from build123d import *

# Parameters (mm, degrees)
SKIZZE1_R                            = 115
AUFSATZ_LINEAR_AUSTRAGEN1_DEPTH      = 730
AUFSATZ_LINEAR_AUSTRAGEN2_DEPTH      = 120
AUFSATZ_LINEAR_AUSTRAGEN2_DEPTH_BACK = 120
SKIZZE2_R                            = 21.686343762


with BuildPart() as part:
    # Skizze1 → Aufsatz-Linear austragen1 (new body)
    with BuildSketch(Plane.XY):
        with Locations(Location((0, 0, 0), (0, 0, 180))):
            Circle(SKIZZE1_R)
    extrude(amount=AUFSATZ_LINEAR_AUSTRAGEN1_DEPTH)

    # Skizze2 → Aufsatz-Linear austragen2 (add, two sides: drawn at the far end of the back side and taken through both)
    with BuildSketch(Plane(origin=(0, 0, 0), x_dir=(1, 0, 0), z_dir=(0, 1, 0)).offset(-AUFSATZ_LINEAR_AUSTRAGEN2_DEPTH_BACK)):
        with Locations(Location((0, -480, 0), (0, 0, 270))):
            Circle(SKIZZE2_R)
    extrude(amount=AUFSATZ_LINEAR_AUSTRAGEN2_DEPTH + AUFSATZ_LINEAR_AUSTRAGEN2_DEPTH_BACK)


solid = part.part
Input: part model. Units: mm. Frame: model coordinates. A direction names the side the tool comes from. Round coordinates to 2 decimals unless told otherwise and drop trailing zeros. Order: outer loops, then holes, each group sorted by start corner. A loop starts at its lowest first (then second) coordinate and runs counter-clockwise, first axis right, second up.
1. Cut plane B-B, the plane x = 0. Output: boundary loops of the cut face in (y, z), then the cut area to 3 significant figures.
The answers:
outline: (-120, 458.31) - (-115, 458.31) - (-115, 0) - (115, 0) - (115, 458.31) - (120, 458.31) - (120, 501.69) - (115, 501.69) - (115, 730) - (-115, 730) - (-115, 501.69) - (-120, 501.69) - close
area: 168,000 mm2
2. Material intervals for line 1 (Y direction, x = -0.5, z = 70); line 2 (Y direction, x = -89, z = 442.5); line 3 (X direction, y = -39, z = 257), sorted ascending.
The answers:
line 1: y = -115 to 115
line 2: y = -72.83 to 72.83
line 3: x = -108.19 to 108.19
3. Cut plane C-C, the plane y = 93. Output: boundary loops of the cut face in (x, z).
The answers:
outline: (-67.65, 0) - (67.65, 0) - (67.65, 730) - (-67.65, 730) - close
4. Set-up query: faces 1 (the face through (18.286, -117.302, 491.658)), 2 (the face through (0, -120, 480)), 3 (the face through (18.286, 117.203, 491.658)). Return all of +Z, -Z, +X, -X, +Y, -Y with unobstructed straight access to the full face (end or side cutting, diameter ignored); none if empty.
The answers:
face 1: -Y
face 2: +Z, -Z, +X, -X, -Y
face 3: +Y
5. Pin query (flat end, axial travel): P1, Ø1, axis at x = -12, z = 414.5, coming from the +Y side; P2, Ø3, axis at x = 61, z = 585, coming from the +Y side; P3, Ø5, axis at x = 19.5, z = 503.5, coming from the -Y side. Return the tip coordinate at first contact, or that it passes through.
The answers:
P1: stops at y = 114.42
P2: stops at y = 98.41
P3: stops at y = -113.74
6. Cut plane A-A, the plane z = 480. Output: boundary loops of the cut face in (x, y), then the cut area to 3 significant figures.
The answers:
outline: (-21.69, -120) - (21.69, -120) - (21.69, -112.94) arc R115 ccw to (21.69, 112.94) - (21.69, 120) - (-21.69, 120) - (-21.69, 112.94) arc R115 ccw to (-21.69, -112.94) - close
area: 42,000 mm2
7. Cut plane D-D, the plane y = 24. Output: boundary loops of the cut face in (x, z), then the cut area to 3 significant figures.
The answers:
outline: (-112.47, 0) - (112.47, 0) - (112.47, 730) - (-112.47, 730) - close
area: 164,000 mm2
